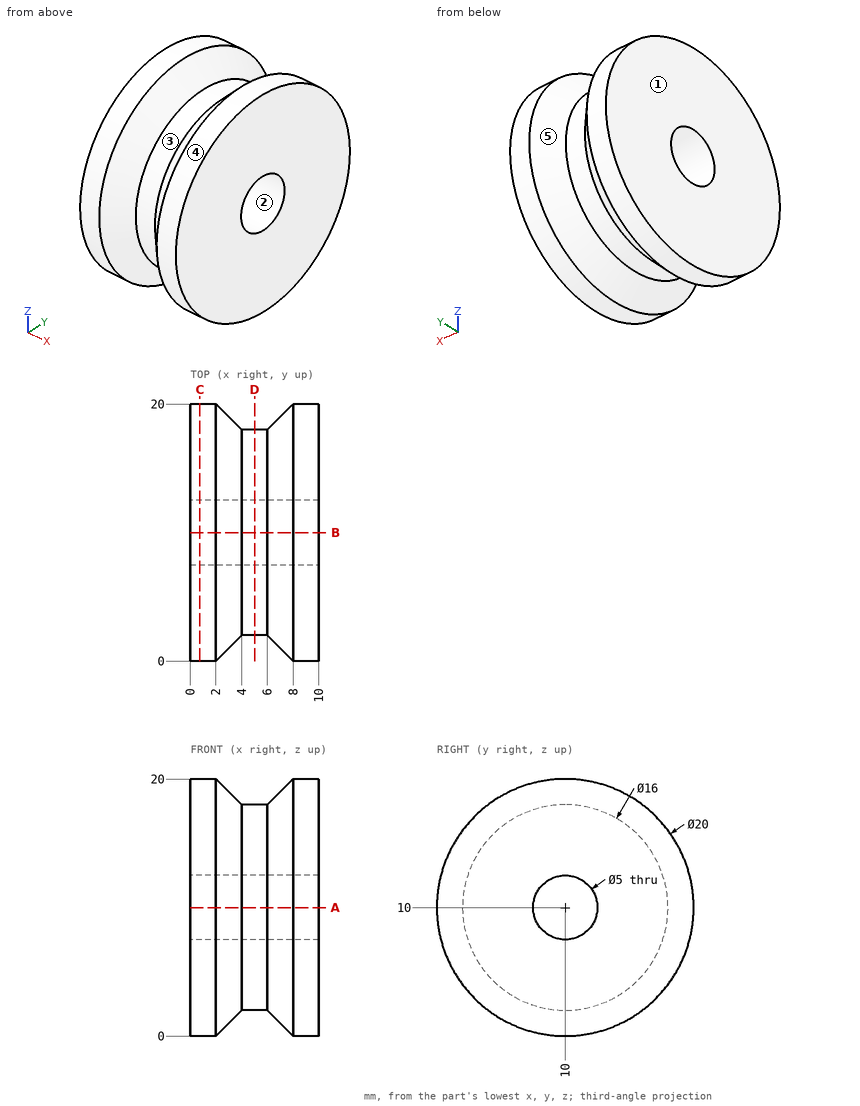
Study the drawing (mm; zero at the part's minimum x, y, z) and answer. A direction names the side the tool comes from. Round coordinates to 2 decimals unless told otherwise and drop trailing zeros. Write each loop counter-clockwise with the first axis right and the second up, starting at its lowest first coordinate (ties: lowest second). Pieces come first, ordered by that corner, then holes.
1) A cutting plane is placed at D-D on x = 5. Determine the outline of the cut face in (y, z), and give its area (3 significant figures).
2) A cutting plane is placed at C-C on x = 0.75. Determine the outline of the cut face in (y, z).
3) Which of the six approach directions +Z, -Z, +X, -X, +Y, -Y give full straight-line access (tool end or side, diameter ignored) to the marked faces 4 and 5?
4) Flat-ended cylindrical pins translate along their axes: P1, Ø1.5, axis at x = 8.5, z = 13.5, coming from the +Y side; P2, Ø5, axis at y = 10, z = 3.5, coming from the -X side; P3, Ø2, axis at x = 2, z = 14, coming from the +Y side. Find the tip coordinate at first contact, or state that the pin passes through.
5) Consider probe 1 along Z at (x, y) = (4.75, 10); probe 2 along Z at (x, y) = (6.5, 10); probe 3 along Y at (x, z) = (5.75, 11). Determine where each line is inside the solid, lowest interval first.
6) A cutting plane is placed at A-A on z = 10. Determine the outline of the cut face in (x, y).
7) Determine the mould class of the marked faces 1, 2 and 3 for opening direction Y: pulls with the +Y half, pulls with the -Y half, needs draft (parallel to the pull), parting line crosses it, or undercut.
Entries:
1. outline: circle Ø16 at (10, 10); hole circle Ø5 at (10, 10)
1. area: 181 mm2
2. outline: circle Ø20 at (10, 10); hole circle Ø5 at (10, 10)
3. face 4: +X, -X
3. face 5: none
4. P1: stops at y = 19.61
4. P2: stops at x = 0
4. P3: stops at y = 19.54
5. probe 1: z = 2 to 7.5, 12.5 to 18
5. probe 2: z = 1.5 to 7.5, 12.5 to 18.5
5. probe 3: y = 2.06 to 7.71, 12.29 to 17.94
6. outline: (0, 0) - (2, 0) - (4, 2) - (6, 2) - (8, 0) - (10, 0) - (10, 7.5) - (0, 7.5) - close; (0, 12.5) - (10, 12.5) - (10, 20) - (8, 20) - (6, 18) - (4, 18) - (2, 20) - (0, 20) - close
7. face 1: needs draft
7. face 2: undercut
7. face 3: parting line crosses it
